The listing builds one solid part. Answer for the finished solid, in the listing's coordinates (mm). A direction names the side the tool comes from. Coordinates: 2 decimals unless noted, no trailing zeros. Order: outer loops, then holes, each group sorted by start corner. A loop starts at its lowest first (then second) coordinate and runs counter-clockwise, first axis right, second up. Notation, with made-up numbers: M 36.25,33.5 L 47.25,33.5 A24 ccw 47.25,66.5 Z; hole C 17.5,79.5 d2. An arc over 180 degrees is marked long. One line per item, written item: value. Start each with the question number.
Q1. Straight lines are drawn through the part: line 1 along Y through (x, z) = (0, 3.75); line 2 along Y through (x, z) = (3, 4.75); line 3 along Y through (x, z) = (4.55, 2.5). For each, find the intervals that lie inside material, in ascending order. Write a range as [from, to].
Q2. For faces 4 (the flat face through (-40, -24, 7)), 5 (the flat face through (0, 42, 3)), 6 (the flat face through (0, -30, 4)), 7 (the flat face through (34.05, -19.82, 5.03)), determine the directions among +Z, -Z, +X, -X, +Y, -Y from which every point of the face is accessible in a straight line to the end or side of a thin tool.
Q3. The part is cut by section A-A on x = -4.55. Give the vertices of the cut face in (y, z).
Q4. Determine the mould class of faces 1 (the flat face through (10, -9, 4)), 2 (the flat face through (8, 13, 8)), 3 (the flat face through (41.632, -23.891, 3.451)) for opening direction X: pulls with the +X half, pulls with the -X half, needs draft (parallel to the pull), parting line crosses it, or undercut.
Q5. Each of these flat-tipped pins is pushed along its axis until it touches: pin 1 Ø3.5 at (x, y) = (3.5, 47) entering from +Z; pin 2 Ø2 at (x, z) = (19, 2.5) entering from -Y; pin 3 Ø2.5 at (y, z) = (15, 7) entering from +X; pin 4 Ø4.5 at (x, y) = (17.5, -6.31) entering from +Z. Where does it stop, or does it pass through?
Q6. The part is cut by section D-D on y = 15. Give the vertices of the cut face in (x, z).
Q7. The part is cut by section B-B on y = 5. Give the vertices of the cut face in (x, z), then the cut area to 3 significant figures.
Q8. The part is cut by section C-C on y = 37.5. Give the vertices of the cut face in (x, z).
```python
from build123d import *

# Parameters (mm, degrees)
BOSS_EXTRUDE1_DEPTH = 8
CUT_EXTRUDE1_DEPTH  = 1
SKETCH3_R           = 1.5
CUT_EXTRUDE2_DEPTH  = 8
SKETCH4_W           = 20
SKETCH4_H           = 5.6
CUT_EXTRUDE3_DEPTH  = 4
SKETCH5_R           = 2.5
SKETCH5_R_2         = 1.5
CUT_EXTRUDE5_DEPTH  = 9
CUT_EXTRUDE6_DEPTH  = 3
FILLET1_R           = 1
FILLET2_R           = 3
FILLET3_R           = 2
FILLET4_R           = 1
FILLET6_R           = 1


with BuildPart() as part:
    # Sketch1 → Boss-Extrude1 (new body)
    with BuildSketch(Plane.XY):
        Polygon((-10, 30.679491924), (-10, 48), (10, 48), (10, 30.679491924), (31.569219382, -6.679491924), (46.569219382, -15.339745962), (36.569219382, -32.660254038), (21.569219382, -24), (16.278513086, -24), (8.795198312, -37), (-8.795198312, -37), (-16.278513086, -24), (-21.569219382, -24), (-36.569219382, -32.660254038), (-46.569219382, -15.339745962), (-31.569219382, -6.679491924), align=None)
    extrude(amount=BOSS_EXTRUDE1_DEPTH)

    # Sketch2 → Cut-Extrude1 (cut)
    with BuildSketch(Plane.XY.offset(8)):
        with BuildLine():
            Line((-36.569219382, -32.660254038), (-46.569219382, -15.339745962))
            Line((-46.569219382, -15.339745962), (-31.846787517, -6.839745962))
            ThreePointArc((-31.846787517, -6.839745962), (-29.570330382, -6.540044695), (-27.748711306, -7.937822174))
            Line((-27.748711306, -7.937822174), (-20.748711306, -20.062177826))
            ThreePointArc((-20.748711306, -20.062177826), (-20.449010038, -22.338634962), (-21.846787517, -24.160254038))
            Line((-21.846787517, -24.160254038), (-36.569219382, -32.660254038))
        make_face()
        with BuildLine():
            Line((-7, 28), (7, 28))
            ThreePointArc((7, 28), (9.121320344, 28.878679656), (10, 31))
            Line((10, 31), (10, 48))
            Line((10, 48), (-10, 48))
            Line((-10, 48), (-10, 31))
            ThreePointArc((-10, 31), (-9.121320344, 28.878679656), (-7, 28))
        make_face()
        with BuildLine():
            Line((36.569219382, -32.660254038), (46.569219382, -15.339745962))
            Line((46.569219382, -15.339745962), (31.846787517, -6.839745962))
            ThreePointArc((31.846787517, -6.839745962), (29.570330382, -6.540044695), (27.748711306, -7.937822174))
            Line((27.748711306, -7.937822174), (20.748711306, -20.062177826))
            ThreePointArc((20.748711306, -20.062177826), (20.449010038, -22.338634962), (21.846787517, -24.160254038))
            Line((21.846787517, -24.160254038), (36.569219382, -32.660254038))
        make_face()
    extrude(amount=-CUT_EXTRUDE1_DEPTH, mode=Mode.SUBTRACT)

    # Sketch3 → Cut-Extrude2 (cut, through all)
    with BuildSketch(Plane.XY.offset(7)):
        with Locations((0, 34)):
            Circle(SKETCH3_R)
        with Locations((29.444863729, -17)):
            Circle(SKETCH3_R)
        with Locations((-29.444863729, -17)):
            Circle(SKETCH3_R)
    extrude(amount=-CUT_EXTRUDE2_DEPTH, mode=Mode.SUBTRACT)

    # Sketch4 → Cut-Extrude3 (cut)
    with BuildSketch(Plane.XY.offset(7)):
        with Locations((0, 42.2)):
            Rectangle(SKETCH4_W, SKETCH4_H)
        Polygon((39.121400909, -11.039745962), (43.97114317, -13.839745962), (33.97114317, -31.160254038), (29.121400909, -28.360254038), align=None)
        Polygon((-43.97114317, -13.839745962), (-39.121400909, -11.039745962), (-29.121400909, -28.360254038), (-33.97114317, -31.160254038), align=None)
    extrude(amount=-CUT_EXTRUDE3_DEPTH, mode=Mode.SUBTRACT)

    # Sketch5 → Cut-Extrude5 (cut, through all)
    with BuildSketch(Plane.XY.offset(8)):
        with Locations((17.5, -6.310889132)):
            Circle(SKETCH5_R)
        with Locations((-4.55, 15)):
            Circle(SKETCH5_R_2)
        with Locations((4.55, -33)):
            Circle(SKETCH5_R_2)
        with BuildLine():
            ThreePointArc((-10, 10), (-9.414213562, 11.414213562), (-8, 12))
            Line((-8, 12), (-1.55, 12))
            Line((-1.55, 12), (1.55, 12))
            Line((1.55, 12), (8, 12))
            ThreePointArc((8, 12), (9.414213562, 11.414213562), (10, 10))
            Line((10, 10), (10, -28))
            ThreePointArc((10, -28), (9.414213562, -29.414213562), (8, -30))
            Line((8, -30), (1.55, -30))
            Line((1.55, -30), (-1.55, -30))
            Line((-1.55, -30), (-8, -30))
            ThreePointArc((-8, -30), (-9.414213562, -29.414213562), (-10, -28))
            Line((-10, -28), (-10, 10))
        make_face()
    extrude(amount=-CUT_EXTRUDE5_DEPTH, mode=Mode.SUBTRACT)

    # Sketch5_3 → Cut-Extrude6 (cut)
    with BuildSketch(Plane.XY.offset(8)):
        with BuildLine():
            Line((1.55, 12), (1.55, 17))
            ThreePointArc((1.55, 17), (0, 18.55), (-1.55, 17))
            Line((-1.55, 17), (-1.55, 12))
            Line((-1.55, 12), (1.55, 12))
        make_face()
        with BuildLine():
            Line((-1.55, -30), (-1.55, -35))
            ThreePointArc((-1.55, -35), (0, -36.55), (1.55, -35))
            Line((1.55, -35), (1.55, -30))
            Line((1.55, -30), (-1.55, -30))
        make_face()
    extrude(amount=-CUT_EXTRUDE6_DEPTH, mode=Mode.SUBTRACT)

    # Fillet1
    fillet1_edges = [part.edges().sort_by_distance(p)[0] for p in [
        (-10, 48, 3.5),
        (10, 48, 3.5),
        (46.569219382, -15.339745962, 3.5),
        (36.569219382, -32.660254038, 3.5),
        (-36.569219382, -32.660254038, 3.5),
        (-46.569219382, -15.339745962, 3.5),
    ]]
    fillet(fillet1_edges, radius=FILLET1_R)

    # Fillet2
    fillet2_edges = [part.edges().sort_by_distance(p)[0] for p in [
        (8.795198312, -37, 4),
        (-8.795198312, -37, 4),
    ]]
    fillet(fillet2_edges, radius=FILLET2_R)

    # Fillet3
    fillet3_edges = [part.edges().sort_by_distance(p)[0] for p in [
        (16.278513086, -24, 4),
        (-16.278513086, -24, 4),
    ]]
    fillet(fillet3_edges, radius=FILLET3_R)

    # Fillet4
    fillet4_edges = [part.edges().sort_by_distance(p)[0] for p in [
        (10, 30.679491924, 4),
    ]]
    fillet(fillet4_edges, radius=FILLET4_R)

    # Fillet6
    fillet6_edges = [part.edges().sort_by_distance(p)[0] for p in [
        (-10, 30.679491924, 4),
    ]]
    fillet(fillet6_edges, radius=FILLET6_R)


solid = part.part
```
Output:
1. line 1: y = [-37, -30], [12, 32.5], [35.5, 39.4], [45, 48]
1. line 2: y = [-37, -30], [12, 39.4], [45, 48]
1. line 3: y = [-37, -34.5], [-31.5, -30], [12, 48]
2. face 4: +Z, -X, +Y, -Y
2. face 5: +Z, +X, -X
2. face 6: +Z, -Z
2. face 7: +Z
3. outline: M -37,0 L -30,0 L -30,8 L -37,8 Z; M 12,0 L 13.5,0 L 13.5,8 L 12,8 Z; M 16.5,0 L 48,0 L 48,7 L 45,7 L 45,3 L 39.4,3 L 39.4,7 L 28,7 L 28,8 L 16.5,8 Z
4. face 1: undercut
4. face 2: needs draft
4. face 3: pulls with the +X half
5. pin 1: stops at z = 7
5. pin 2: stops at y = -24
5. pin 3: stops at x = 19.77
5. pin 4: passes through
6. outline: M -19.05,0 L -6.05,0 L -6.05,8 L -19.05,8 Z; M -3.05,0 L 19.05,0 L 19.05,8 L 1.55,8 L 1.55,5 L -1.55,5 L -1.55,8 L -3.05,8 Z
7. outline: M -24.83,0 L -10,0 L -10,8 L -24.83,8 Z; M 10,0 L 24.83,0 L 24.83,8 L 10,8 Z
7. area: 237 mm^2
8. outline: M -10,0 L 10,0 L 10,7 L -10,7 Z
